Autodesk Inventor part; units mm, degrees
ref_plane "Work Plane1" through (0, 0, 0) normal (0, 0, 1) x (1, 0, 0)
ref_plane "YZ Plane" through (0, 0, 0) normal (1, 0, 0) x (0, 1, 0)
ref_plane "XZ Plane" through (0, 0, 0) normal (0, 1, 0) x (-1, 0, 0)
sketch "Sketch1" plane through (0, 0, 0) normal (1, 0, 0) x (0, 1, 0)
  circle A0 centre (0, 0) radius 12.5
  dimension "d0" = 25
extrude "Extrusion1" add sketch "Sketch1" along normal blind 8
sketch "Sketch2" plane through (8, 0, 0) normal (1, 0, 0) x (0, 0, -1)
  circle A0 centre (0, 0) radius 6
  dimension "d3" = 12
extrude "Extrusion2" cut sketch "Sketch2" against normal blind 8
thread "Thread1"
sketch "Sketch3" plane through (8, 0, 0) normal (1, 0, 0) x (0, 0, -1)
  circle A0 centre (0, 0) radius 12.5
  line L0 (0, 12.5) -> (0, 10.5)
  line L1 (0, 10.5) -> (-2, 10.5)
  line L2 (-2, 10.5) -> (2, 10.5)
  line L3 (-2, 10.5) -> (-2, 12.339)
  line L4 (-2, 13.4004) -> (2, 13.4004)
  line L5 (2, 13.4004) -> (2, 10.5)
  line L6 (-2, 12.339) -> (-2, 13.4004)
  line L7 (-12.5, 0) -> (-10.5, 0)
  line L8 (-10.5, 0) -> (-10.5, -2)
  line L9 (-10.5, -2) -> (-10.5, 2)
  line L10 (-10.5, -2) -> (-12.339, -2)
  line L11 (-13.4004, -2) -> (-13.4004, 2)
  line L12 (-13.4004, 2) -> (-10.5, 2)
  line L13 (-12.339, -2) -> (-13.4004, -2)
  line L14 (0, -12.5) -> (0, -10.5)
  line L15 (0, -10.5) -> (2, -10.5)
  line L16 (2, -10.5) -> (-2, -10.5)
  line L17 (2, -10.5) -> (2, -12.339)
  line L18 (2, -13.4004) -> (-2, -13.4004)
  line L19 (-2, -13.4004) -> (-2, -10.5)
  line L20 (2, -12.339) -> (2, -13.4004)
  line L21 (12.5, 0) -> (10.5, 0)
  line L22 (10.5, 0) -> (10.5, 2)
  line L23 (10.5, 2) -> (10.5, -2)
  line L24 (10.5, 2) -> (12.339, 2)
  line L25 (13.4004, 2) -> (13.4004, -2)
  line L26 (13.4004, -2) -> (10.5, -2)
  line L27 (12.339, 2) -> (13.4004, 2)
  dimension "d9" = 2
  dimension "d10" = 4
  dimension "d16" = 360
extrude "Extrusion3" cut sketch "Sketch3" against normal blind 8 contours L21 L22 L24 A0 | A0 L27 L25 L26 | A0 L26 L23 L21 | L5 L2 L0 A0 | A0 L6 L4 L5 | L20 L18 L19 A0 | A0 L14 L15 L17 | L0 L1 L3 A0 | A0 L19 L16 L14 | L12 L9 L7 A0 | A0 L13 L11 L12 | A0 L7 L8 L10
ref_plane "Work Plane1" through (0, 0, 0) normal (0, 0, 1) x (1, 0, 0)
properties part number "7. LockNutM12" material "Lead"
Verification items for the finished model (mm, model axes). A direction names the side the tool comes from. Round coordinates to 2 decimals unless told otherwise and drop trailing zeros. Write each loop counter-clockwise with the first axis right and the second up, starting at its lowest first coordinate (ties: lowest second). Pieces come first, ordered by that corner, then holes.
(1) Section check D-D (z = -8.5). Enter the section's corners in (x, y), plus the area to 3 significant figures.
Returned:
outline: (0, -9.17) - (8, -9.17) - (8, 9.17) - (0, 9.17) - close
area: 147 mm2
(2) Section check C-C (x = 6.25). Enter the section's corners in (y, z), plus the area to 3 significant figures.
Returned:
outline: (-12.34, -2) arc R12.5 ccw to (-2, -12.34) - (-2, -10.5) - (2, -10.5) - (2, -12.34) arc R12.5 ccw to (12.34, -2) - (10.5, -2) - (10.5, 2) - (12.34, 2) arc R12.5 ccw to (2, 12.34) - (2, 10.5) - (-2, 10.5) - (-2, 12.34) arc R12.5 ccw to (-12.34, 2) - (-10.5, 2) - (-10.5, -2) - close; hole circle Ø12 at (0, 0)
area: 347 mm2
(3) Section check A-A (y = 0). Enter the section's corners in (x, z), plus the area to 3 significant figures.
Returned:
outline: (0, -10.5) - (8, -10.5) - (8, -6) - (0, -6) - close; (0, 6) - (8, 6) - (8, 10.5) - (0, 10.5) - close
area: 72.0 mm2
(4) Access from +Z, -Z, +X, -X, +Y, -Y to the whole of each face (thin tool, end or side, straight path). Record for faces 1 (the flat face through (4, 0, 10.5)), 2 (the flat face through (4, -10.5, 0)), 3 (the flat face through (4, 2, -11)), 4 (the flat face through (4, 10.5, 0)), 5 (the cylindrical face through (3.944, 8.916, -8.761)).
Returned:
face 1: +Z, +X, -X
face 2: +X, -X, -Y
face 3: -Z, +X, -X
face 4: +X, -X, +Y
face 5: -Z, +X, -X, +Y
(5) Material ranges on line 1 (Y direction, x = 3.75, z = 0); line 2 (Z direction, x = 6.75, y = 3.75); line 3 (Y direction, x = 4.5, z = 4.75), recorded low to high.
Returned:
line 1: y = -10.5 to -6, 6 to 10.5
line 2: z = -11.92 to -4.68, 4.68 to 11.92
line 3: y = -11.56 to -3.67, 3.67 to 11.56
(6) Mould release check, pull along Z, two halves, no side actions. Record for faces 6 (the cylindrical face through (3.944, -8.761, -8.916)), 7 (the flat face through (0, -6, 3)), 8 (the flat face through (4, 11, -2)): pulls with the +Z half, pulls with the -Z half, needs draft (parallel to the pull), parting line crosses it, or undercut.
Returned:
face 6: pulls with the -Z half
face 7: needs draft
face 8: undercut
(7) Depth check by flat-ended pin: pin 1 Ø2 at (x, y) = (2.5, 11.5) entering from +Z; pin 2 Ø1.5 at (x, y) = (3, 11.5) entering from -Z; pin 3 Ø2 at (x, y) = (4.5, 0.5) entering from +Z; pin 4 Ø2 at (y, z) = (-9, 4) entering from -X. Enter the tip coordinate at first touch or a pass-through.
Returned:
pin 1: stops at z = 6.78
pin 2: stops at z = -6.38
pin 3: stops at z = 10.5
pin 4: stops at x = 0
